Input: dimensioned drawing with shaded views. Units: mm. Origin: part minimum x, y, z. A direction names the side the tool comes from. Round coordinates to 2 decimals unless told otherwise and drop trailing zeros. Write each loop counter-clockwise with the first axis right and the second up, starting at its lowest first coordinate (ties: lowest second). Pieces come first, ordered by that corner, then holes. Notation, with made-up numbers: (5.5, 17) -> (29.5, 17) arc R11 ccw to (29.5, 36) -> close; hole circle Ø2 at (-1, 87.5). An arc over 180 degrees is marked (long way). Use one line per item in the form item = value. Start each with the question number.
1. Reachability of the marked faces 4, 5 and 6 from +Z, -Z, +X, -X, +Y, -Y: full face, straight path, thin tool, end or side. Return the list, or none.
2. Draft query along Z for the marked faces 1, 2 and 3. Return one class per face: pulls with the +Z half, pulls with the -Z half, needs draft (parallel to the pull), parting line crosses it, or undercut.
3. Cut plane D-D, the plane z = 23.75. Return the cut outline in (x, y), plus the area to 3 significant figures.
4. Pin query (flat end, axial travel): pin 1 Ø2 at (x, z) = (5, 4) entering from +Y; pin 2 Ø6.5 at (x, y) = (4.5, 11.5) entering from -Z; pin 3 Ø6 at (x, y) = (12, 8) entering from +Z; pin 4 Ø5 at (x, z) = (10.5, 22.5) entering from +Y. Return the tip coordinate at first contact, or that it passes through.
5. Cut plane B-B, the plane z = 15.25. Return the cut outline in (x, y).
6. Cut plane C-C, the plane x = 7.75. Return the cut outline in (y, z).
7. Cut plane A-A, the plane y = 4.5. Return the cut outline in (x, z).
8. Line query: L1, parallel to Z at x = 7.75, y = 1.25; L2, parallel to X at y = 11.25, z = 19.5; L3, parallel to Y at x = 6.25, z = 6.5. Output: solid intervals per line, ascending.
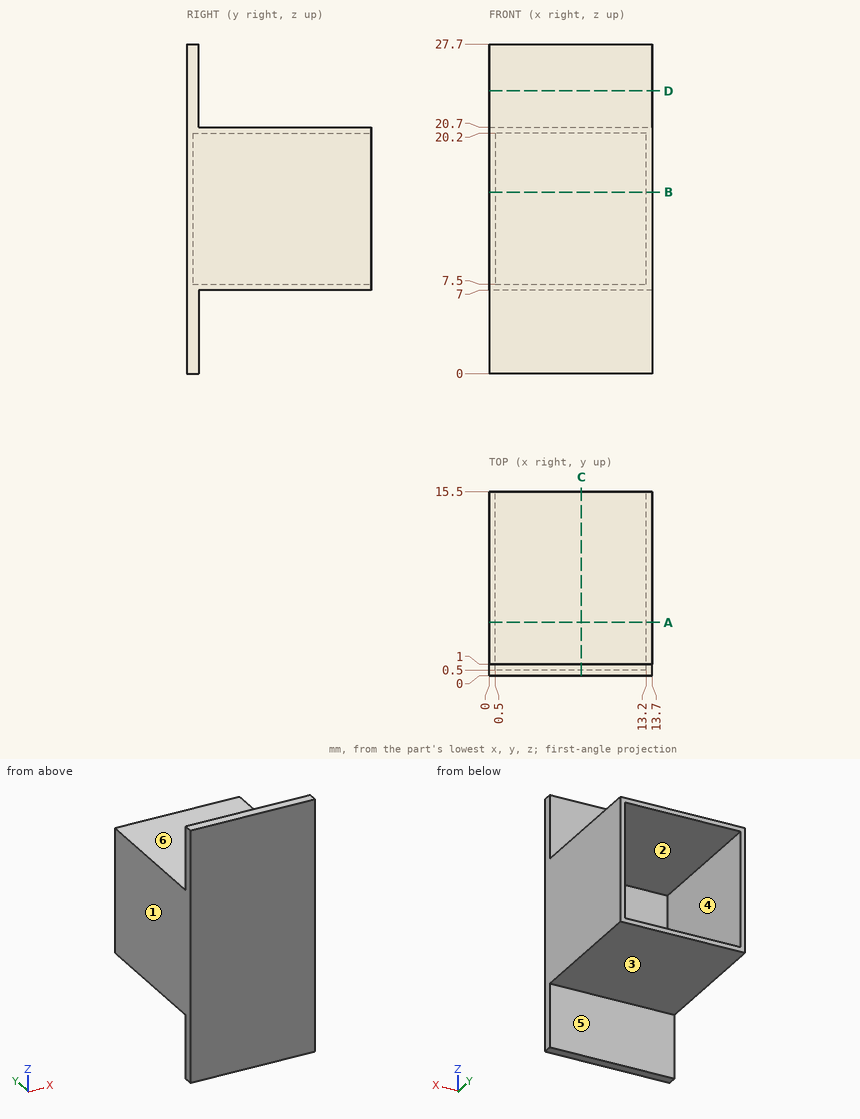
Outcome:
q1.face_4 = +Y
q1.face_5 = -Z, +X, -X, +Y
q1.face_6 = +Z, +X, -X, +Y
q2.face_1 = needs draft
q2.face_2 = undercut
q2.face_3 = pulls with the -Z half
q3.outline = (0, 0) -> (13.7, 0) -> (13.7, 1) -> (0, 1) -> close
q3.area = 13.7 mm^2
q4.pin_1 = 1
q4.pin_2 = 7
q4.pin_3 = 20.7
q4.pin_4 = 15.5
q5.outline = (0, 0) -> (13.7, 0) -> (13.7, 15.5) -> (13.2, 15.5) -> (13.2, 0.5) -> (0.5, 0.5) -> (0.5, 15.5) -> (0, 15.5) -> close
q6.outline = (0, 0) -> (1, 0) -> (1, 7) -> (15.5, 7) -> (15.5, 7.5) -> (0.5, 7.5) -> (0.5, 20.2) -> (15.5, 20.2) -> (15.5, 20.7) -> (1, 20.7) -> (1, 27.7) -> (0, 27.7) -> close
q7.outline = (0, 7) -> (13.7, 7) -> (13.7, 20.7) -> (0, 20.7) -> close; hole (0.5, 7.5) -> (13.2, 7.5) -> (13.2, 20.2) -> (0.5, 20.2) -> close
q8.L1 = 7 to 7.5, 20.2 to 20.7
q8.L2 = 0 to 0.5, 13.2 to 13.7
q8.L3 = 0 to 1
